Design review of the part built by this model. Coordinates are the model's own, in mm. Give positions to 0.01 mm unless a question says otherwise; leave off trailing zeros. Loops run counter-clockwise (first coordinate to the right, second up) from the corner with the lowest first, then second, coordinate; pieces in that order, holes last.
from build123d import *

# Parameters (mm, degrees)
F0_R     = 4
F1_DEPTH = 12.7


# Not quite as in the source:
# - a feature names something its author has since deleted; it is built from what else it names


with BuildPart() as f1:
    # F0 (on Front) → F1 (new body)
    with BuildSketch(Plane.XZ):
        with BuildLine():
            ThreePointArc((-50.8, -9), (-44.4360389693, -6.3639610307), (-41.8, 0))
            ThreePointArc((-41.8, 0), (-44.4360389693, 6.3639610307), (-50.8, 9))
            ThreePointArc((-50.8, 9), (-59.8, 0), (-50.8, -9))
        make_face()
        with Locations((-50.8, 0)):
            Circle(F0_R, mode=Mode.SUBTRACT)
        with BuildLine():
            ThreePointArc((9, 0), (6.3639610238, 6.3639610375), (-1.93e-08, 9))
            ThreePointArc((-1.93e-08, 9), (-9, -9.7e-09), (0, -9))
            ThreePointArc((0, -9), (6.3639610307, -6.3639610307), (9, 0))
        make_face()
        Circle(F0_R, mode=Mode.SUBTRACT)
        with BuildLine():
            ThreePointArc((-50.8, 9), (-44.4360389693, 6.3639610307), (-41.8, 0))
            ThreePointArc((-41.8, 0), (-44.4360389693, -6.3639610307), (-50.8, -9))
            Line((-50.8, -9), (0, -9))
            ThreePointArc((0, -9), (-9, -9.7e-09), (-1.93e-08, 9))
            Line((-1.93e-08, 9), (-50.8, 9))
        make_face()
        with BuildLine():
            Line((44.45, 9), (-1.93e-08, 9))
            ThreePointArc((-1.93e-08, 9), (6.3639610238, 6.3639610375), (9, 0))
            ThreePointArc((9, 0), (6.3639610307, -6.3639610307), (0, -9))
            Line((0, -9), (44.45, -9))
            ThreePointArc((44.45, -9), (35.45, 0), (44.45, 9))
        make_face()
        with BuildLine():
            ThreePointArc((53.45, 0), (50.8139610307, 6.3639610307), (44.45, 9))
            ThreePointArc((44.45, 9), (35.45, 0), (44.45, -9))
            ThreePointArc((44.45, -9), (50.8139610307, -6.3639610307), (53.45, 0))
        make_face()
        with Locations((44.45, 0)):
            Circle(F0_R, mode=Mode.SUBTRACT)
    extrude(amount=F1_DEPTH)


solid = f1.part
Q1. Draft analysis for pull direction X (two halves, no side actions). For faces 1 (the face through (-3, -6, 9)), 2 (the face through (48.265, -6.261, 1.201)), 3 (the face through (-59.798, -6.261, 0.198)), state which applies: pulls with the +X half, pulls with the -X half, needs draft (parallel to the pull), parting line crosses it, or undercut.
Results:
face 1: needs draft
face 2: undercut
face 3: pulls with the -X half
Q2. Take a section at D-D (z = -7.25). Give the boundary of the cut face in (x, y).
Results:
outline: (-56.13, -12.7) - (49.78, -12.7) - (49.78, 0) - (-56.13, 0) - close
Q3. Insertion check: pin 1 (5 mm diameter, centred on x = 0, z = 0, fed in from +Y). The pin has a flat end and moves straight along its axis. Give the tip position at first contact, or say it passes through.
Results:
pin 1: passes through
Q4. Take a section at A-A (y = -11). Give the boundary of the cut face in (x, z), plus the area to 3 significant figures.
Results:
outline: (-50.8, -9) - (44.45, -9) arc R9 ccw to (44.45, 9) - (-50.8, 9) arc R9 ccw to start; hole circle Ø8 at (-50.8, 0); hole circle Ø8 at (0, 0); hole circle Ø8 at (44.45, 0)
area: 1,820 mm2
Q5. Wall thickness on line 1 (X direction, y = -6.75, z = -1); line 2 (X direction, y = -1.25, z = 3.25); line 3 (Z direction, x = 0, y = -7): over which ranges is each line inside the solid? List them lowest first.
Results:
line 1: x = -59.74 to -54.67, -46.93 to -3.87, 3.87 to 40.58, 48.32 to 53.39
line 2: x = -59.19 to -53.13, -48.47 to -2.33, 2.33 to 42.12, 46.78 to 52.84
line 3: z = -9 to -4, 4 to 9
Q6. Take a section at C-C (x = -49). Give the boundary of the cut face in (y, z).
Results:
outline: (-12.7, -9) - (0, -9) - (0, -3.57) - (-12.7, -3.57) - close; (-12.7, 3.57) - (0, 3.57) - (0, 9) - (-12.7, 9) - close
Q7. Take a section at B-B (x = 0). Give the boundary of the cut face in (y, z).
Results:
outline: (-12.7, -9) - (0, -9) - (0, -4) - (-12.7, -4) - close; (-12.7, 4) - (0, 4) - (0, 9) - (-12.7, 9) - close
